Can you work these out from the model? Positions are in its coordinate system, mm. Coordinates: 2 decimals unless noted, no trailing zeros. Order: outer loops, then holes, each group sorted by start corner. A loop starts at its lowest first (then second) coordinate and runs counter-clockwise, first axis right, second up. Notation, with made-up numbers: (78, -24) -> (124, -24) arc R10 cw to (124, -15) -> close; hole circle Ø11 at (19.25, -15.75). An arc over 180 degrees is marked (long way). Write item = value, one per line. Start each with the question number.
from build123d import *

# Parameters (mm, degrees)
SKETCH_1_R      = 1.6
SKETCH_1_R_2    = 4
EXTRUDE_1_DEPTH = 3


with BuildPart() as part:
    # 草图1 → 凸台-拉伸1 (new body)
    with BuildSketch(Plane(origin=(0, 0, 0), x_dir=(1, 0, 0), z_dir=(0, 1, 0))):
        with BuildLine():
            Line((5, 75), (-5, 75))
            ThreePointArc((-5, 75), (-8.535533906, 73.535533906), (-10, 70))
            Line((-10, 70), (-10, 65))
            ThreePointArc((-10, 65), (-11.464466094, 61.464466094), (-15, 60))
            Line((-15, 60), (-36, 60))
            ThreePointArc((-36, 60), (-43.071067812, 62.928932188), (-46, 70))
            Line((-46, 70), (-46, 145))
            ThreePointArc((-46, 145), (-44.535533906, 148.535533906), (-41, 150))
            Line((-41, 150), (-35, 150))
            ThreePointArc((-35, 150), (-31.464466094, 148.535533906), (-30, 145))
            Line((-30, 145), (-30, 135))
            Line((-30, 135), (30, 135))
            Line((30, 135), (30, 145))
            ThreePointArc((30, 145), (31.464466094, 148.535533906), (35, 150))
            Line((35, 150), (41, 150))
            ThreePointArc((41, 150), (44.535533906, 148.535533906), (46, 145))
            Line((46, 145), (46, 70))
            ThreePointArc((46, 70), (43.071067812, 62.928932188), (36, 60))
            Line((36, 60), (15, 60))
            ThreePointArc((15, 60), (11.464466094, 61.464466094), (10, 65))
            Line((10, 65), (10, 70))
            ThreePointArc((10, 70), (8.535533906, 73.535533906), (5, 75))
        make_face()
        with Locations(Location((-40, 118, 0), (0, 0, 270))):
            Circle(SKETCH_1_R, mode=Mode.SUBTRACT)
        with Locations(Location((40, 129, 0), (0, 0, 270))):
            Circle(SKETCH_1_R, mode=Mode.SUBTRACT)
        with Locations(Location((-40, 129, 0), (0, 0, 270))):
            Circle(SKETCH_1_R, mode=Mode.SUBTRACT)
        with Locations(Location((40, 118, 0), (0, 0, 270))):
            Circle(SKETCH_1_R, mode=Mode.SUBTRACT)
        with Locations(Location((-16.5, 83, 0), (0, 0, 270))):
            Circle(SKETCH_1_R, mode=Mode.SUBTRACT)
        with Locations(Location((16.5, 83, 0), (0, 0, 270))):
            Circle(SKETCH_1_R, mode=Mode.SUBTRACT)
        with Locations(Location((-25, 130.5, 0), (0, 0, 270))):
            Circle(SKETCH_1_R, mode=Mode.SUBTRACT)
        with Locations(Location((25, 130.5, 0), (0, 0, 270))):
            Circle(SKETCH_1_R, mode=Mode.SUBTRACT)
        with Locations(Location((-16.5, 130, 0), (0, 0, 270))):
            Circle(SKETCH_1_R, mode=Mode.SUBTRACT)
        with Locations(Location((16.5, 130, 0), (0, 0, 270))):
            Circle(SKETCH_1_R, mode=Mode.SUBTRACT)
        with Locations(Location((0, 118, 0), (0, 0, 270))):
            Circle(SKETCH_1_R, mode=Mode.SUBTRACT)
        with Locations(Location((0, 93, 0), (0, 0, 270))):
            Circle(SKETCH_1_R, mode=Mode.SUBTRACT)
        with Locations(Location((-29, 105.5, 0), (0, 0, 270))):
            Circle(SKETCH_1_R_2, mode=Mode.SUBTRACT)
        with Locations(Location((-29, 97.5, 0), (0, 0, 270))):
            Circle(SKETCH_1_R, mode=Mode.SUBTRACT)
        with Locations(Location((-29, 113.5, 0), (0, 0, 270))):
            Circle(SKETCH_1_R, mode=Mode.SUBTRACT)
        with Locations(Location((-19.5, 105.5, 0), (0, 0, 270))):
            Circle(SKETCH_1_R, mode=Mode.SUBTRACT)
        with Locations(Location((-38.5, 105.5, 0), (0, 0, 270))):
            Circle(SKETCH_1_R, mode=Mode.SUBTRACT)
        with Locations(Location((38.5, 105.5, 0), (0, 0, 270))):
            Circle(SKETCH_1_R, mode=Mode.SUBTRACT)
        with Locations(Location((19.5, 105.5, 0), (0, 0, 270))):
            Circle(SKETCH_1_R, mode=Mode.SUBTRACT)
        with Locations(Location((29, 113.5, 0), (0, 0, 270))):
            Circle(SKETCH_1_R, mode=Mode.SUBTRACT)
        with Locations(Location((29, 97.5, 0), (0, 0, 270))):
            Circle(SKETCH_1_R, mode=Mode.SUBTRACT)
        with Locations(Location((29, 105.5, 0), (0, 0, 270))):
            Circle(SKETCH_1_R_2, mode=Mode.SUBTRACT)
        with Locations(Location((40, 140, 0), (0, 0, 270))):
            Circle(SKETCH_1_R, mode=Mode.SUBTRACT)
        with Locations(Location((-40, 140, 0), (0, 0, 270))):
            Circle(SKETCH_1_R, mode=Mode.SUBTRACT)
        with BuildLine():
            Line((36, 78), (36, 80))
            ThreePointArc((36, 80), (34.535533906, 83.535533906), (31, 85))
            Line((31, 85), (25, 85))
            ThreePointArc((25, 85), (21.464466094, 83.535533906), (20, 80))
            Line((20, 80), (20, 78))
            ThreePointArc((20, 78), (21.464466094, 74.464466094), (25, 73))
            Line((25, 73), (31, 73))
            ThreePointArc((31, 73), (34.535533906, 74.464466094), (36, 78))
        make_face(mode=Mode.SUBTRACT)
        with BuildLine():
            Line((-25, 85), (-31, 85))
            ThreePointArc((-31, 85), (-34.535533906, 83.535533906), (-36, 80))
            Line((-36, 80), (-36, 78))
            ThreePointArc((-36, 78), (-34.535533906, 74.464466094), (-31, 73))
            Line((-31, 73), (-25, 73))
            ThreePointArc((-25, 73), (-21.464466094, 74.464466094), (-20, 78))
            Line((-20, 78), (-20, 80))
            ThreePointArc((-20, 80), (-21.464466094, 83.535533906), (-25, 85))
        make_face(mode=Mode.SUBTRACT)
    extrude(amount=EXTRUDE_1_DEPTH)


solid = part.part
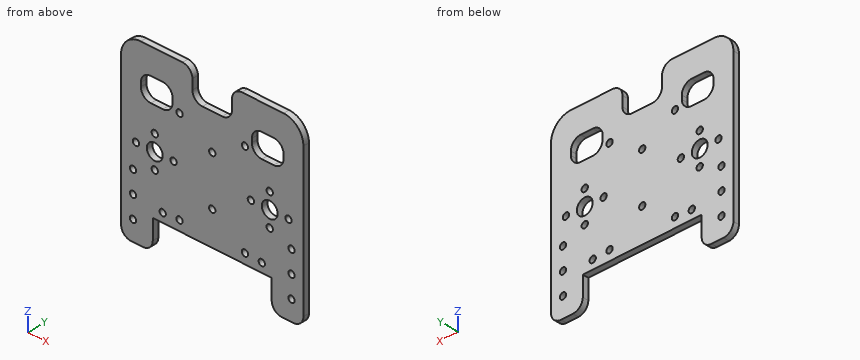
(1) Imagine slicing it at A-A (x = 0). Write out the boundary of the cut face in (y, z).
(2) Imagine slicing it at D-D (y = 2). Count the separate pieces of the cut face and the enclosed holes in it, plus the area to 3 significant figures.
(3) Imagine slicing it at B-B (z = -105.5). Write out the boundary of the cut face in (x, y), plus the area to 3 significant figures.
(4) If I drill on L1, parallel to X at y = 1.8, z = -113.5; L2, parallel to Z at x = 17.5, y = 2.8; L3, parallel to X at y = 2.55, z = -74, over which ranges is the centre line in solid material (lowest first)? Write a range as from..to.
(5) Imagine slicing it at C-C (z = -71.5). Write out the boundary of the cut face in (x, y).
(6) For P1, Ø1.5, axis at x = 28, y = 2, coming from the -Z side; P2, Ø1.5, axis at y = 1.5, z = -68.5, coming from the +X side, each with a flat end and sliding along its axis, tell me the tip position at first contact or that it passes through.
Result set:
q1.outline = (0, -135) -> (3, -135) -> (3, -119.6) -> (0, -119.6) -> close; (0, -116.4) -> (3, -116.4) -> (3, -94.6) -> (0, -94.6) -> close; (0, -91.4) -> (3, -91.4) -> (3, -75) -> (0, -75) -> close
q2.separate_pieces = 1
q2.enclosed_holes = 26
q2.area = 6,400 mm2
q3.outline = (-46, 0) -> (-40.1, 0) -> (-40.1, 3) -> (-46, 3) -> close; (-36.9, 0) -> (-33, 0) -> (-33, 3) -> (-36.9, 3) -> close; (-25, 0) -> (-21.1, 0) -> (-21.1, 3) -> (-25, 3) -> close; (-17.9, 0) -> (17.9, 0) -> (17.9, 3) -> (-17.9, 3) -> close; (21.1, 0) -> (25, 0) -> (25, 3) -> (21.1, 3) -> close; (33, 0) -> (36.9, 0) -> (36.9, 3) -> (33, 3) -> close; (40.1, 0) -> (46, 0) -> (46, 3) -> (40.1, 3) -> close
q3.area = 190 mm2
q4.L1 = -46..-30.6, -27.4..27.4, 30.6..46
q4.L2 = -135..-131.25, -128.75..-84.25, -81.75..-60
q4.L3 = -46..-34, -22..-8, 8..22, 34..46
q5.outline = (-46, 0) -> (-9.77, 0) -> (-9.77, 3) -> (-46, 3) -> close; (9.77, 0) -> (46, 0) -> (46, 3) -> (9.77, 3) -> close
q6.P1 = -135
q6.P2 = 45.97
